from build123d import *

# Parameters (mm, degrees)
SKETCH1_R           = 10
BOSS_EXTRUDE1_DEPTH = 25
SKETCH2_R           = 4
CUT_EXTRUDE1_DEPTH  = 10
SKETCH3_R           = 2.5
CUT_EXTRUDE2_DEPTH  = 10
CHAMFER1_SIZE       = 0.5


with BuildPart() as part:
    # Sketch1 → Boss-Extrude1 (new body)
    with BuildSketch(Plane(origin=(0, 0, 0), x_dir=(1, 0, 0), z_dir=(0, 1, 0))):
        with Locations(Location((0, 0, 0), (0, 0, 270))):
            Circle(SKETCH1_R)
    extrude(amount=BOSS_EXTRUDE1_DEPTH)

    # Sketch2 → Cut-Extrude1 (cut)
    with BuildSketch(Plane(origin=(0, 25, 0), x_dir=(1, 0, 0), z_dir=(0, 1, 0))):
        with Locations(Location((0, 0, 0), (0, 0, 270))):
            Circle(SKETCH2_R)
    extrude(amount=-CUT_EXTRUDE1_DEPTH, mode=Mode.SUBTRACT)

    # Sketch3 → Cut-Extrude2 (cut)
    with BuildSketch(Plane.XZ):
        with Locations(Location((0, 0, 0), (0, 0, 270))):
            Circle(SKETCH3_R)
    extrude(amount=-CUT_EXTRUDE2_DEPTH, mode=Mode.SUBTRACT)

    # Chamfer1
    chamfer1_edges = [part.edges().sort_by_distance(p)[0] for p in [
        (0, 0, 2.5),
        (0, 0, -10),
        (0, 25, -10),
        (0, 25, -4),
    ]]
    chamfer(chamfer1_edges, length=CHAMFER1_SIZE)


solid = part.part
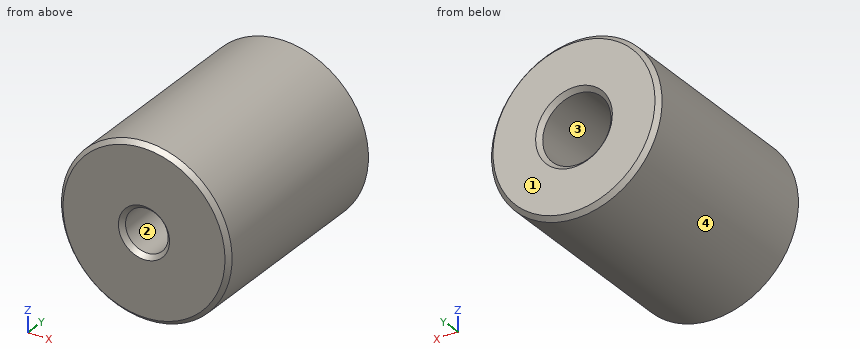
The model under review builds one solid part; all positions refer to its coordinate system, in mm. Face numbers are marked on the shaded views. Coordinates: 2 decimals unless noted, no trailing zeros. Loops run counter-clockwise (first coordinate to the right, second up) from the corner with the lowest first, then second, coordinate; pieces in that order, holes last.
(1) Consider section A-A, the plane x = 0. Give the boundary of the cut face in (y, z).
Determined:
outline: (0, -9.5) - (0.5, -10) - (24.5, -10) - (25, -9.5) - (25, -4.5) - (24.5, -4) - (15, -4) - (15, 4) - (24.5, 4) - (25, 4.5) - (25, 9.5) - (24.5, 10) - (0.5, 10) - (0, 9.5) - (0, 3) - (0.5, 2.5) - (10, 2.5) - (10, -2.5) - (0.5, -2.5) - (0, -3) - close
(2) Insertion check: P1, Ø1.5, axis at x = 6.5, y = 12.5, coming from the +Z side; P2, Ø3, axis at x = 0, z = 0, coming from the -Y side; P3, Ø2, axis at y = 17.5, z = 6.5, coming from the -X side. Each pin has a flat end and moves straight along its axis. Give the tip position at first contact, or say it passes through.
Determined:
P1: stops at z = 8.18
P2: stops at y = 10
P3: stops at x = -8.35
(3) Consider section D-D, the plane y = 13.25. Give the boundary of the cut face in (x, z), plus the area to 3 significant figures.
Determined:
outline: circle Ø20 at (0, 0)
area: 314 mm2
(4) Draft analysis for pull direction X (two halves, no side actions). For the marked faces 1, 2, 3 and 4, state which applies: +X half, -X half, draft (parallel to the pull), parting line (faces both ways), or undercut.
Determined:
face 1: draft
face 2: undercut
face 3: undercut
face 4: parting line
(5) Consider section B-B, the plane z = 0. Give the boundary of the cut face in (x, y), plus the area to 3 significant figures.
Determined:
outline: (-10, 0.5) - (-9.5, 0) - (-3, 0) - (-2.5, 0.5) - (-2.5, 10) - (2.5, 10) - (2.5, 0.5) - (3, 0) - (9.5, 0) - (10, 0.5) - (10, 24.5) - (9.5, 25) - (4.5, 25) - (4, 24.5) - (4, 15) - (-4, 15) - (-4, 24.5) - (-4.5, 25) - (-9.5, 25) - (-10, 24.5) - close
area: 369 mm2
(6) Consider section C-C, the plane y = 20.5. Give the boundary of the cut face in (x, z).
Determined:
outline: circle Ø20 at (0, 0); hole circle Ø8 at (0, 0)
(7) Wall thickness on L1, parallel to X at y = 18.75, z = 0; L2, parallel to X at y = 2.5, z = 0; L3, parallel to Y at x = 1.5, z = 0.5: over which ranges is each line inside the solid? List them lowest first.
Determined:
L1: x = -10 to -4, 4 to 10
L2: x = -10 to -2.5, 2.5 to 10
L3: y = 10 to 15
